For this review, use the dimensioned drawing (mm, ordinates from the lowest corner) and the shaded views. A direction names the side the tool comes from. Coordinates: 2 decimals unless noted, no trailing zeros. Loops run counter-clockwise (first coordinate to the right, second up) from the corner with the lowest first, then second, coordinate; pieces in that order, holes last. Notation, with made-up numbers: M 24,47 L 77,47 A28 ccw 77,80 Z; hole C 68,66 d7. An arc over 180 degrees is marked long. One line per item, written item: value.
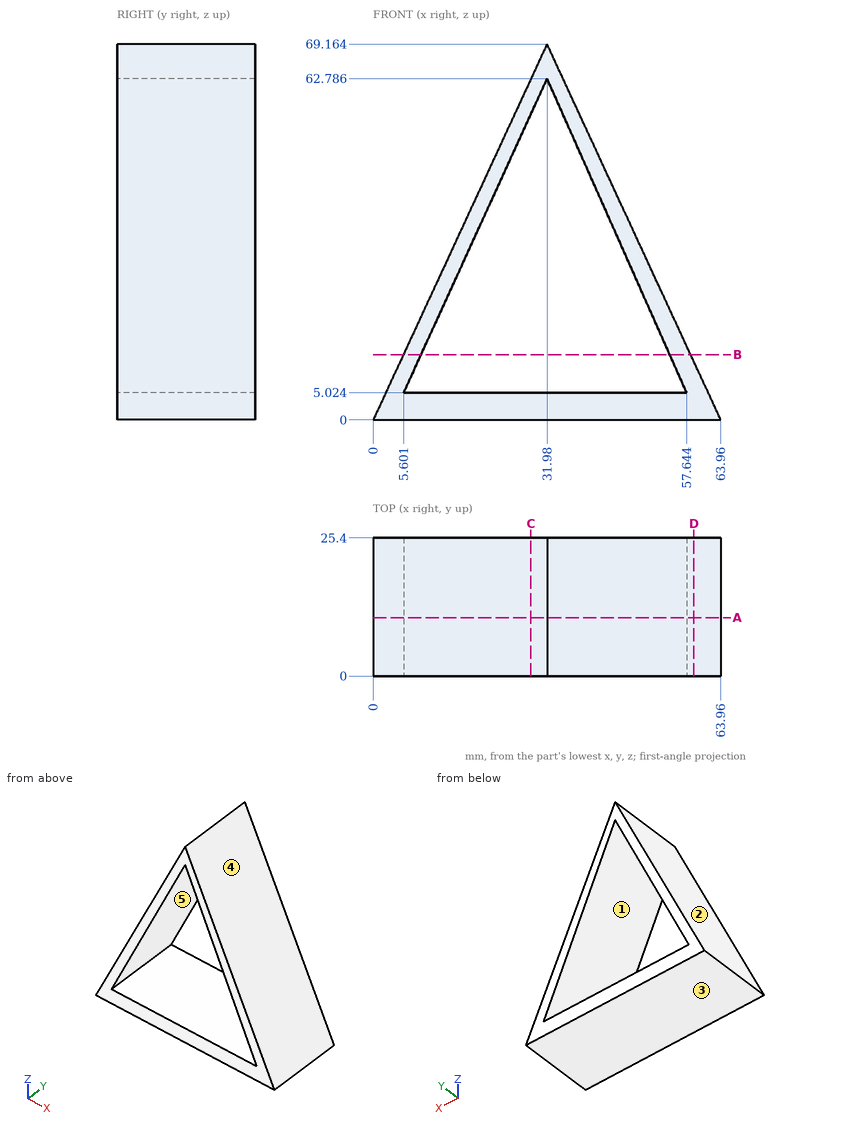
(1) Add section C-C on x = 29. State the section outline as (y, z) points.
Checks:
outline: M 0,0 L 25.4,0 L 25.4,5.02 L 0,5.02 Z; M 0,56.26 L 25.4,56.26 L 25.4,62.72 L 0,62.72 Z
(2) To check wall thickness, follow L1, parallel to Z at x = 43, y = 13.5 (1 decimal); L2, parallel to X at y = 13.75, z = 60; L3, parallel to Z at x = 47.5, y = 3.25 (1 decimal). State the ranges of each line that lie inside material, in increasing order. Write a range as [from, to].
Checks:
L1: [0, 5], [38, 45.3]
L2: [27.74, 30.71], [33.22, 36.22]
L3: [0, 5], [27.9, 35.6]
(3) Insertion check: pin 1 Ø7.5 at (x, y) = (37.5, 15) entering from +Z (1 decimal); pin 2 Ø3 at (y, z) = (5, 13.5) entering from -X; pin 3 Ø6 at (y, z) = (17.5, 30) entering from +X (1 decimal); pin 4 Ø12 at (x, y) = (36.5, 13.5) entering from -Z. Each pin has a flat end and moves straight along its axis. Give the tip position at first contact, or say it passes through.
Checks:
pin 1: z = 65.3
pin 2: x = 5.55
pin 3: x = 51.5
pin 4: z = 0
(4) Draft analysis for pull direction Z (two halves, no side actions). For the marked faces 3, 4 and 5, state which applies: pulls with the +Z half, pulls with the -Z half, needs draft (parallel to the pull), parting line crosses it, or undercut.
Checks:
face 3: pulls with the -Z half
face 4: pulls with the +Z half
face 5: undercut
(5) Add section A-A on y = 10.75. State the section outline as (x, z) points (1 decimal), then the cut area to 3 significant figures.
Checks:
outline: M 0,0 L 64,0 L 32,69.2 Z; hole M 5.6,5 L 57.6,5 L 32,62.8 Z
area: 709 mm^2
(6) Add section B-B on z = 12. State the section outline as (x, y) points (1 decimal).
Checks:
outline: M 5.5,0 L 8.8,0 L 8.8,25.4 L 5.5,25.4 Z; M 54.5,0 L 58.4,0 L 58.4,25.4 L 54.5,25.4 Z
(7) Add section D-D on x = 59. State the section outline as (y, z) points.
Checks:
outline: M 0,0 L 25.4,0 L 25.4,10.73 L 0,10.73 Z
(8) Tool access review of the marked faces 1 and 2: name each direction out of +Z, -Z, +X, -X, +Y, -Y from which nothing blocks a thin tool from reaching the whole face with its end or side.
Checks:
face 1: +Y, -Y
face 2: +Z, -X, +Y, -Y
